Here's how the part is built. I have some questions about the finished solid (model axes, mm). Face numbers are marked on the shaded views. A direction names the side the tool comes from. Round coordinates to 2 decimals unless told otherwise and drop trailing zeros. Loops run counter-clockwise (first coordinate to the right, second up) from the corner with the lowest first, then second, coordinate; pieces in that order, holes last. Notation, with made-up numbers: M 29,59.5 L 53,59.5 A20 cw 53,98.5 Z; hole C 80.5,12 d9. An arc over 180 degrees is marked long. Answer as a JSON object with one key per item and string values.
from build123d import *

# Parameters (mm, degrees)
SKETCH1_W           = 240
SKETCH1_H           = 50
BOSS_EXTRUDE1_DEPTH = 25
SKETCH1_5_W         = 240
SKETCH1_5_H         = 50
CUT_EXTRUDE1_DEPTH  = 20
BOSS_EXTRUDE3_START = -25
SKETCH1_6_W         = 10
SKETCH1_6_H         = 10
SKETCH1_6_R         = 2
BOSS_EXTRUDE3_DEPTH = 5
BOSS_EXTRUDE4_START = 25
BOSS_EXTRUDE4_DEPTH = 5
SKETCH2_W           = 15
SKETCH2_H           = 15
SKETCH2_R           = 5
BOSS_EXTRUDE5_DEPTH = 5
FILLET1_R           = 2.5


with BuildPart() as part:
    # Sketch1 → Boss-Extrude1 (new, symmetric)
    with BuildSketch(Plane.XY):
        Polygon((-125, 30), (-125, -30), (125, -30), (125, 30), (120, 30), (120, 25), (120, -25), (-120, -25), (-120, 25), (-120, 30), align=None)
        Rectangle(SKETCH1_W, SKETCH1_H)
        Polygon((-55, 30), (-120, 30), (-120, 25), (120, 25), (120, 30), (57.5, 30), (55, 30), (45, 30), (42.5, 30), (-45, 30), align=None)
    extrude(amount=BOSS_EXTRUDE1_DEPTH, both=True)

    # Sketch1<5> → Cut-Extrude1 (cut, symmetric)
    with BuildSketch(Plane.XY):
        Rectangle(SKETCH1_5_W, SKETCH1_5_H)
        Polygon((-55, 30), (-120, 30), (-120, 25), (120, 25), (120, 30), (57.5, 30), (55, 30), (45, 30), (42.5, 30), (-45, 30), align=None)
    extrude(amount=CUT_EXTRUDE1_DEPTH, both=True, mode=Mode.SUBTRACT)

    # Sketch1<6> → Boss-Extrude3 (add)
    with BuildSketch(Plane.XY.offset(BOSS_EXTRUDE3_START)):
        with Locations((-50, 35)):
            Rectangle(SKETCH1_6_W, SKETCH1_6_H)
        with Locations((-50, 35)):
            Circle(SKETCH1_6_R, mode=Mode.SUBTRACT)
        with Locations((50, 35)):
            Rectangle(SKETCH1_6_W, SKETCH1_6_H)
        with Locations((50, 35)):
            Circle(SKETCH1_6_R, mode=Mode.SUBTRACT)
    extrude(amount=BOSS_EXTRUDE3_DEPTH)

    # Sketch1<8> → Boss-Extrude4 (add)
    with BuildSketch(Plane.XY.offset(BOSS_EXTRUDE4_START)):
        with BuildLine():
            Line((45, 30), (55, 30))
            Line((55, 30), (55, 37.5))
            ThreePointArc((55, 37.5), (50, 32.5), (45, 37.5))
            Line((45, 37.5), (45, 30))
        make_face()
        with BuildLine():
            Line((55, 30), (57.5, 30))
            Line((57.5, 30), (57.5, 45))
            Line((57.5, 45), (42.5, 45))
            Line((42.5, 45), (42.5, 30))
            Line((42.5, 30), (45, 30))
            Line((45, 30), (45, 37.5))
            Line((45, 37.5), (45, 40))
            Line((45, 40), (45.669872981, 40))
            ThreePointArc((45.669872981, 40), (50, 42.5), (54.330127019, 40))
            Line((54.330127019, 40), (55, 40))
            Line((55, 40), (55, 37.5))
            Line((55, 37.5), (55, 30))
        make_face()
        with BuildLine():
            Line((45, 40), (45, 37.5))
            ThreePointArc((45, 37.5), (45.170370869, 38.794095226), (45.669872981, 40))
            Line((45.669872981, 40), (45, 40))
        make_face()
        with BuildLine():
            ThreePointArc((54.330127019, 40), (54.829629131, 38.794095226), (55, 37.5))
            Line((55, 37.5), (55, 40))
            Line((55, 40), (54.330127019, 40))
        make_face()
    extrude(amount=-BOSS_EXTRUDE4_DEPTH)

    # Sketch2 → Boss-Extrude5 (add)
    with BuildSketch(Plane.ZY.offset(125)):
        with Locations((0, 37.5)):
            Rectangle(SKETCH2_W, SKETCH2_H)
        with Locations((0, 37.5)):
            Circle(SKETCH2_R, mode=Mode.SUBTRACT)
    extrude(amount=-BOSS_EXTRUDE5_DEPTH)

    # Fillet1
    fillet1_edges = [part.edges().sort_by_distance(p)[0] for p in [
        (-41.25, 30, 25),
        (125, 30, 0),
        (-125, 0, 25),
        (0, -30, 25),
        (0, 30, -25),
        (-45, 40, -22.5),
        (-55, 40, -22.5),
        (90, 30, -25),
        (55, 40, -22.5),
        (125, 0, 25),
        (45, 40, -22.5),
        (0, -30, -25),
        (91.25, 30, 25),
        (-125, 0, -25),
        (57.5, 45, 22.5),
        (42.5, 45, 22.5),
        (-90, 30, -25),
        (125, 0, -25),
        (-125, 30, -16.25),
        (-122.5, 45, 7.5),
        (-122.5, 45, -7.5),
        (125, -30, 0),
        (-125, -30, 0),
        (-125, 30, 16.25),
    ]]
    fillet(fillet1_edges, radius=FILLET1_R)


solid = part.part
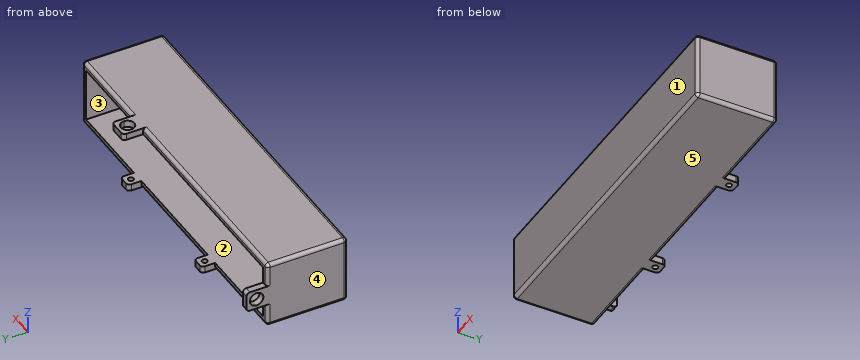
Item 1: On a 3-axis mill with a long thin cutter (end or side, diameter ignored), from which of +Z, -Z, +X, -X, +Y, -Y can I reach the whole of each face in a straight line? I mean the marked faces 1 and 2. Say none if no direction works.
Resolved:
{"face 1": "+Z, -Z, +X, -X, -Y", "face 2": "+Y"}
Item 2: I want a section at B-B, the plane x = -27. Please give me the cut outline in (y, z), then the cut area to 3 significant figures.
Resolved:
{"outline": "M -30,-22.5 A2.5 ccw -27.5,-25 L 27.5,-25 A2.5 ccw 30,-22.5 L 30,-20 L -25,-20 L -25,20 L 30,20 L 30,22.5 A2.5 ccw 27.5,25 L -27.5,25 A2.5 ccw -30,22.5 Z", "area": "795 mm²"}
Item 3: I'm going to push flat-ended pins straight in: pin 1 Ø11.5 at (y, z) = (37.5, 0) entering from +X; pin 2 Ø12 at (x, z) = (-93, 0.5) entering from +Y; pin 3 Ø1.5 at (x, y) = (-123, 36) entering from +Z. Where does each tip first touch, or does it pass through?
Resolved:
{"pin 1": "x = -120", "pin 2": "y = -25", "pin 3": "z = 7.5"}
Item 4: I want a section at C-C, the plane y = 2.5. Please give me the cut outline in (x, z), then the cut area to 3 significant figures.
Resolved:
{"outline": "M -125,-22.5 A2.5 ccw -122.5,-25 L 122.5,-25 A2.5 ccw 125,-22.5 L 125,22.5 A2.5 ccw 122.5,25 L -122.5,25 A2.5 ccw -125,22.5 Z; hole M -120,-20 L 120,-20 L 120,20 L -120,20 Z", "area": "2,890 mm²"}
Item 5: I want a section at D-D, the plane z = 0. Please give me the cut outline in (x, y), then the cut area to 3 significant figures.
Resolved:
{"outline": "M -125,-27.5 A2.5 ccw -122.5,-30 L 122.5,-30 A2.5 ccw 125,-27.5 L 125,27.5 A2.5 ccw 122.5,30 L 120,30 L 120,-25 L -120,-25 L -120,32.5 L -125,32.5 Z; M -125,42.5 L -120,42.5 L -120,45 L -125,45 Z", "area": "1,820 mm²"}
Item 6: I want a section at A-A, the plane z = -13. Please give me the cut outline in (x, y), then the cut area to 3 significant figures.
Resolved:
{"outline": "M -125,-27.5 A2.5 ccw -122.5,-30 L 122.5,-30 A2.5 ccw 125,-27.5 L 125,27.5 A2.5 ccw 122.5,30 L 120,30 L 120,-25 L -120,-25 L -120,30 L -122.5,30 A2.5 ccw -125,27.5 Z", "area": "1,790 mm²"}
Item 7: Please list where these lines run through material, in increasing order: probe 1 along X at (y, z) = (4.5, -9); probe 2 along Z at (x, y) = (-32.5, 12); probe 3 along Y at (x, z) = (-121, 0). Write a range as from..to.
Resolved:
{"probe 1": "-125..-120, 120..125", "probe 2": "-25..-20, 20..25", "probe 3": "-30..32.5, 42.5..45"}
Item 8: If we mould it in two halves opening along X, with no side actions, what happens to the marked faces 3, 4 and 5? For each: pulls with the +X half, pulls with the -X half, needs draft (parallel to the pull), parting line crosses it, or undercut.
Resolved:
{"face 3": "undercut", "face 4": "pulls with the -X half", "face 5": "needs draft"}
